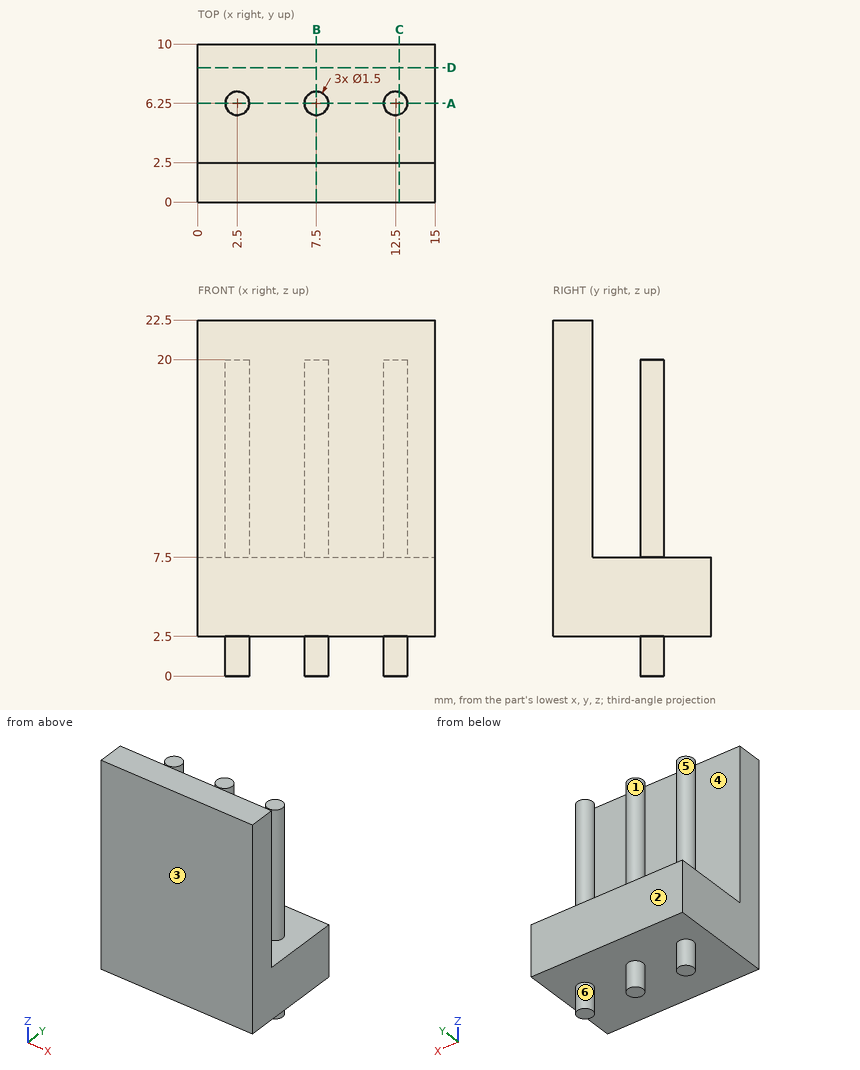
Verification items for this drawing (mm, ordinates from the low corner). A direction names the side the tool comes from. Coordinates: 2 decimals unless noted, no trailing zeros. Loops run counter-clockwise (first coordinate to the right, second up) from the corner with the lowest first, then second, coordinate; pieces in that order, holes last.
Item 1: Go/stop test with flat-tipped pins: pin 1 Ø1.6 at (x, y) = (12.5, 6.5) entering from +Z; pin 2 Ø4 at (x, z) = (5, 11) entering from +Y. Record where each tip stops, or that it passes through.
Item 2: Sectioned sample at C-C, the plane x = 12.75. Record the boundary of the cut face in (y, z).
Item 3: Sectioned sample at B-B, the plane x = 7.5. Record the boundary of the cut face in (y, z).
Item 4: Access from +Z, -Z, +X, -X, +Y, -Y to the whole of each face (thin tool, end or side, straight path). Record for the marked faces 4, 5 and 6.
Item 5: Sectioned sample at A-A, the plane y = 6.25. Record the boundary of the cut face in (x, z).
Item 6: Thickness scan on line 1 (Y direction, x = 7.5, z = 9.5); line 2 (X direction, y = 6, z = 2); line 3 (Z direction, x = 12.25, y = 6.25). Record the ranges inside material, lowest first.
Item 7: Release check for a two-part mould opening along Y. For the marked faces 1, 2 and 3 record: released by +Y, released by -Y, zero draft, split by the parting line, or undercut.
Item 8: Sectioned sample at D-D, the plane y = 8.5. Record the boundary of the cut face in (x, z), then the cut area to 3 significant figures.
Check result:
1. pin 1: stops at z = 20
1. pin 2: stops at y = 6.81
2. outline: (0, 2.5) - (5.54, 2.5) - (5.54, 0) - (6.96, 0) - (6.96, 2.5) - (10, 2.5) - (10, 7.5) - (6.96, 7.5) - (6.96, 20) - (5.54, 20) - (5.54, 7.5) - (2.5, 7.5) - (2.5, 22.5) - (0, 22.5) - close
3. outline: (0, 2.5) - (5.5, 2.5) - (5.5, 0) - (7, 0) - (7, 2.5) - (10, 2.5) - (10, 7.5) - (7, 7.5) - (7, 20) - (5.5, 20) - (5.5, 7.5) - (2.5, 7.5) - (2.5, 22.5) - (0, 22.5) - close
4. face 4: +Z, +X, -X
4. face 5: +Z
4. face 6: -Z
5. outline: (0, 2.5) - (1.75, 2.5) - (1.75, 0) - (3.25, 0) - (3.25, 2.5) - (6.75, 2.5) - (6.75, 0) - (8.25, 0) - (8.25, 2.5) - (11.75, 2.5) - (11.75, 0) - (13.25, 0) - (13.25, 2.5) - (15, 2.5) - (15, 7.5) - (13.25, 7.5) - (13.25, 20) - (11.75, 20) - (11.75, 7.5) - (8.25, 7.5) - (8.25, 20) - (6.75, 20) - (6.75, 7.5) - (3.25, 7.5) - (3.25, 20) - (1.75, 20) - (1.75, 7.5) - (0, 7.5) - close
6. line 1: y = 0 to 2.5, 5.5 to 7
6. line 2: x = 1.79 to 3.21, 6.79 to 8.21, 11.79 to 13.21
6. line 3: z = 0 to 20
7. face 1: undercut
7. face 2: released by +Y
7. face 3: released by -Y
8. outline: (0, 2.5) - (15, 2.5) - (15, 7.5) - (0, 7.5) - close
8. area: 75.0 mm2
